```python
from build123d import *

# Parameters (mm, degrees)
SKETCH1_R           = 1.5
BOSS_EXTRUDE1_DEPTH = 1.75
BOSS_DEPTH          = 3
BOSS_EXTRUDE5_DEPTH = 1.5
SKETCH10_R          = 0.25
CUT_EXTRUDE2_DEPTH  = 5.5


with BuildPart() as part:
    # Sketch1 → Boss-Extrude1 (new body)
    with BuildSketch(Plane(origin=(0, 0, 0), x_dir=(1, 0, 0), z_dir=(0, 1, 0))):
        with BuildLine():
            Line((-16, -18), (16, -18))
            ThreePointArc((16, -18), (17.414213562, -17.414213562), (18, -16))
            Line((18, -16), (18, 16))
            ThreePointArc((18, 16), (17.414213562, 17.414213562), (16, 18))
            Line((16, 18), (-16, 18))
            ThreePointArc((-16, 18), (-17.414213562, 17.414213562), (-18, 16))
            Line((-18, 16), (-18, -16))
            ThreePointArc((-18, -16), (-17.414213562, -17.414213562), (-16, -18))
        make_face()
        with Locations((-15.25, 15.25)):
            Circle(SKETCH1_R, mode=Mode.SUBTRACT)
        with Locations((15.25, 15.25)):
            Circle(SKETCH1_R, mode=Mode.SUBTRACT)
        with Locations((-15.25, -15.25)):
            Circle(SKETCH1_R, mode=Mode.SUBTRACT)
        with Locations((15.25, -15.25)):
            Circle(SKETCH1_R, mode=Mode.SUBTRACT)
    extrude(amount=BOSS_EXTRUDE1_DEPTH)

    # Sketch2 → Boss- (add)
    with BuildSketch(Plane.XY.offset(18)):
        with BuildLine():
            Line((4.683071404, 1.75), (8.659974309, 1.75))
            Line((8.659974309, 1.75), (8.659974309, 3.094003243))
            ThreePointArc((8.659974309, 3.094003243), (8.601395665, 3.235424599), (8.459974309, 3.294003243))
            Line((8.459974309, 3.294003243), (8.281537536, 3.294003243))
            ThreePointArc((8.281537536, 3.294003243), (8.14011618, 3.352581887), (8.081537536, 3.494003243))
            Line((8.081537536, 3.494003243), (8.081537536, 3.55))
            ThreePointArc((8.081537536, 3.55), (8.022958893, 3.691421356), (7.881537536, 3.75))
            Line((7.881537536, 3.75), (5.461508176, 3.75))
            ThreePointArc((5.461508176, 3.75), (5.32008682, 3.691421356), (5.261508176, 3.55))
            Line((5.261508176, 3.55), (5.261508176, 3.494003243))
            ThreePointArc((5.261508176, 3.494003243), (5.202929533, 3.352581887), (5.061508176, 3.294003243))
            Line((5.061508176, 3.294003243), (4.883071404, 3.294003243))
            ThreePointArc((4.883071404, 3.294003243), (4.741650048, 3.235424599), (4.683071404, 3.094003243))
            Line((4.683071404, 3.094003243), (4.683071404, 1.75))
        make_face()
        with BuildLine():
            Line((4.783071404, 1.85), (4.783071404, 3.094003243))
            ThreePointArc((4.783071404, 3.094003243), (4.812360726, 3.164713921), (4.883071404, 3.194003243))
            Line((4.883071404, 3.194003243), (5.061508176, 3.194003243))
            ThreePointArc((5.061508176, 3.194003243), (5.273640211, 3.281871209), (5.361508176, 3.494003243))
            Line((5.361508176, 3.494003243), (5.361508176, 3.55))
            ThreePointArc((5.361508176, 3.55), (5.390797498, 3.620710678), (5.461508176, 3.65))
            Line((5.461508176, 3.65), (7.881537536, 3.65))
            ThreePointArc((7.881537536, 3.65), (7.952248214, 3.620710678), (7.981537536, 3.55))
            Line((7.981537536, 3.55), (7.981537536, 3.494003243))
            ThreePointArc((7.981537536, 3.494003243), (8.069405502, 3.281871209), (8.281537536, 3.194003243))
            Line((8.281537536, 3.194003243), (8.459974309, 3.194003243))
            ThreePointArc((8.459974309, 3.194003243), (8.530684987, 3.164713921), (8.559974309, 3.094003243))
            Line((8.559974309, 3.094003243), (8.559974309, 1.85))
            Line((8.559974309, 1.85), (4.783071404, 1.85))
        make_face(mode=Mode.SUBTRACT)
    extrude(amount=-BOSS_DEPTH)

    # Sketch9 → Boss-Extrude5 (add)
    with BuildSketch(Plane(origin=(0, 0, 15), x_dir=(-1, 0, 0), z_dir=(0, 0, -1))):
        with BuildLine():
            Line((-8.281537536, 3.294003243), (-8.459974309, 3.294003243))
            ThreePointArc((-8.459974309, 3.294003243), (-8.601395665, 3.235424599), (-8.659974309, 3.094003243))
            Line((-8.659974309, 3.094003243), (-8.659974309, 1.75))
            Line((-8.659974309, 1.75), (-4.683071404, 1.75))
            Line((-4.683071404, 1.75), (-4.683071404, 3.094003243))
            ThreePointArc((-4.683071404, 3.094003243), (-4.741650048, 3.235424599), (-4.883071404, 3.294003243))
            Line((-4.883071404, 3.294003243), (-5.061508176, 3.294003243))
            ThreePointArc((-5.061508176, 3.294003243), (-5.202929533, 3.352581887), (-5.261508176, 3.494003243))
            Line((-5.261508176, 3.494003243), (-5.261508176, 3.55))
            ThreePointArc((-5.261508176, 3.55), (-5.32008682, 3.691421356), (-5.461508176, 3.75))
            Line((-5.461508176, 3.75), (-7.881537536, 3.75))
            ThreePointArc((-7.881537536, 3.75), (-8.022958893, 3.691421356), (-8.081537536, 3.55))
            Line((-8.081537536, 3.55), (-8.081537536, 3.494003243))
            ThreePointArc((-8.081537536, 3.494003243), (-8.14011618, 3.352581887), (-8.281537536, 3.294003243))
        make_face()
    extrude(amount=BOSS_EXTRUDE5_DEPTH)

    # Sketch10 → Cut-Extrude2 (cut, through all)
    with BuildSketch(Plane(origin=(0, 0, 13.5), x_dir=(-1, 0, 0), z_dir=(0, 0, -1))):
        with Locations((-6.686931658, 2.562814542)):
            Circle(SKETCH10_R)
        with Locations((-5.886931658, 2.562814542)):
            Circle(SKETCH10_R)
        with Locations((-7.486931658, 2.562814542)):
            Circle(SKETCH10_R)
    extrude(amount=-CUT_EXTRUDE2_DEPTH, mode=Mode.SUBTRACT)


solid = part.part
```
Source: CAD feature listing. Evaluate the final solid. Frame: model axes, mm. A direction names the side the tool comes from. Round coordinates to 2 decimals unless told otherwise and drop trailing zeros. Loops run counter-clockwise (first coordinate to the right, second up) from the corner with the lowest first, then second, coordinate; pieces in that order, holes last. Notation, with made-up numbers: M -12,70 L 47,70 A12 ccw 47,91 Z; hole C -6,15.25 d5. An arc over 180 degrees is marked long. Use a Markdown table: item, result. Add a question column.
1. Cut plane D-D, the plane z = 4.5. Output: boundary loops of the cut face in (x, y), and give its area (3 significant figures).
2. Cut plane B-B, the plane z = -15.25. Output: boundary loops of the cut face in (x, y).
3. Cut plane C-C, the plane y = 0.85. Output: boundary loops of the cut face in (x, z), and give its area (3 significant figures).
4. Contact query for flat-ended pins moving along their axis: pin 1 (2 mm diameter, centred on x = -5.5, y = 2, fed in from +Z); pin 2 (0.5 mm diameter, centred on x = 6.5, y = 3, fed in from +Z); pin 3 (5 mm diameter, centred on x = 4, z = -13, fed in from +Y); pin 4 (1 mm diameter, centred on y = 2.5, z = 16.5, fed in from -X). Output: stop coordinate, or through.
5. Set-up query: faces 1 (the flat face through (7, 3, 15)), 2 (the cylindrical face through (-16.75, 0.86, -15.32)), 3 (the flat face through (7, 3, 13.5)). Return all of +Z, -Z, +X, -X, +Y, -Y with unobstructed straight access to the full face (end or side cutting, diameter ignored); none if empty.
6. Cut plane A-A, the plane x = -15.25. Output: boundary loops of the cut face in (y, z), and give its area (3 significant figures).
7. Pull-direction query (X, two-part tool) for faces 4 (the cylindrical face through (17.4, 0.86, 17.43)), 5 (the flat face through (0, 0, 0)), 6 (the cylindrical face through (-16.75, 0.86, 15.18)), 7 (the flat face through (7, 1.85, 17)); classes: +X half, -X half, draft (parallel to the pull), parting line (faces both ways), or undercut.
8. Ray query, line 1 along X through (y, z) = (1.25, 15.25); line 2 along X through (y, z) = (2.45, 14). Return the intervals inside material, ascending. Write a range as [from, to].
Solution:
| question | item | result |
|---|---|---|
| 1 | outline | M -18,0 L 18,0 L 18,1.75 L -18,1.75 Z |
| 1 | area | 63.0 mm2 |
| 2 | outline | M -18,0 L -16.75,0 L -16.75,1.75 L -18,1.75 Z; M -13.75,0 L 13.75,0 L 13.75,1.75 L -13.75,1.75 Z; M 16.75,0 L 18,0 L 18,1.75 L 16.75,1.75 Z |
| 3 | outline | M -18,-16 A2 ccw -16,-18 L 16,-18 A2 ccw 18,-16 L 18,16 A2 ccw 16,18 L -16,18 A2 ccw -18,16 Z; hole C -15.25,-15.25 d3; hole C -15.25,15.25 d3; hole C 15.25,-15.25 d3; hole C 15.25,15.25 d3 |
| 3 | area | 1,260 mm2 |
| 4 | pin 1 | stops at z = 18 |
| 4 | pin 2 | stops at z = 15 |
| 4 | pin 3 | stops at y = 1.75 |
| 4 | pin 4 | stops at x = 4.68 |
| 5 | face 1 | +Z |
| 5 | face 2 | +Y, -Y |
| 5 | face 3 | -Z, +X, -X, +Y |
| 6 | outline | M 0,-18 L 1.75,-18 L 1.75,-16.75 L 0,-16.75 Z; M 0,-13.75 L 1.75,-13.75 L 1.75,13.75 L 0,13.75 Z; M 0,16.75 L 1.75,16.75 L 1.75,18 L 0,18 Z |
| 6 | area | 52.5 mm2 |
| 7 | face 4 | +X half |
| 7 | face 5 | draft |
| 7 | face 6 | undercut |
| 7 | face 7 | undercut |
| 8 | line 1 | x = [-18, -16.75], [-13.75, 13.75], [16.75, 18] |
| 8 | line 2 | x = [4.68, 5.66], [6.11, 6.46], [6.91, 7.26], [7.71, 8.66] |
